Model file for the job. Use its own axes, mm. A direction names the side the tool comes from. Give positions to 0.01 mm unless a question says otherwise; leave off trailing zeros. Order: outer loops, then holes, each group sorted by start corner. A loop starts at its lowest first (then second) coordinate and runs counter-clockwise, first axis right, second up. Notation, with made-up numbers: (38, 48) - (68, 48) arc R13 cw to (68, 72) - close; hole circle Ø2 at (-27.5, 35). An arc over 180 degrees is marked (long way). Use CSV: the item, a comma, the result in double quotes. Start each with the question number.
(1) Probe L1, parallel to Z at x = 34.8, y = -4.25; L2, parallel to X at y = -2, z = 34. List the from-to ranges inside material, lowest first.
(2) Band-saw the part on B-B, the plane y = -56. Give the cut face in (x, z), then the cut area to 3 significant figures.
(3) Band-saw the part on A-A, the plane x = -34.8. Give the cut face in (y, z), then the cut area to 3 significant figures.
(4) Drop flat-ended pins along their axis: pin 1 Ø3 at (x, y) = (6, 28) entering from +Z; pin 2 Ø5.5 at (y, z) = (-56, 36) entering from +X; pin 3 Ø16 at (x, z) = (38, -38) entering from -Y. Give the stop position or say it passes through.
(5) Tool access for faces 1 (the flat face through (27.9, -45, -35)), 2 (the flat face through (-35, -45, -27.9)), 3 (the cylindrical face through (26.4, -44.51, 41.47)), 4 (the flat face through (-39, 0, 1)), 5 (the cylindrical face through (-26.4, -44.51, 41.47)): list every direction of +Z, -Z, +X, -X, +Y, -Y with a clear straight run to the whole face (end or side of a thin tool).
(6) Band-saw the part on C-C, the plane x = 0. Give the cut face in (y, z).
(7) Band-saw the part on D-D, the plane z = 34.8. Give the cut face in (x, y), then the cut area to 3 significant figures.
from build123d import *

# Parameters (mm, degrees)
F1_DEPTH  = 80
F2_W      = 15
F2_H      = 15
F3_DEPTH  = 70
F4_R      = 3.25
F5_DEPTH  = 10
F6_R      = 5
F7_R      = 36.5
F8_DEPTH  = 1.6
F9_R      = 7
F10_DEPTH = 35
F13_DEPTH = 5


with BuildPart() as f1:
    # F0 (on Front) → F1 (new body)
    with BuildSketch(Plane.XZ):
        with BuildLine():
            Line((37.9, 42.9), (-37.9, 42.9))
            ThreePointArc((-37.9, 42.9), (-41.4355339059, 41.4355339059), (-42.9, 37.9))
            Line((-42.9, 37.9), (-42.9, -37.9))
            ThreePointArc((-42.9, -37.9), (-41.4355339059, -41.4355339059), (-37.9, -42.9))
            Line((-37.9, -42.9), (37.9, -42.9))
            ThreePointArc((37.9, -42.9), (41.4355339059, -41.4355339059), (42.9, -37.9))
            Line((42.9, -37.9), (42.9, 37.9))
            ThreePointArc((42.9, 37.9), (41.4355339059, 41.4355339059), (37.9, 42.9))
        make_face()
    extrude(amount=F1_DEPTH)

    # F2 (on face) → F3 (cut)
    with BuildSketch(Plane.XZ.offset(80)):
        with Locations((35.4, 35.4)):
            Rectangle(F2_W, F2_H)
        with Locations((-35.4, 35.4)):
            Rectangle(F2_W, F2_H)
        with Locations((-35.4, -35.4)):
            Rectangle(F2_W, F2_H)
        with Locations((35.4, -35.4)):
            Rectangle(F2_W, F2_H)
    extrude(amount=-F3_DEPTH, mode=Mode.SUBTRACT)

    # F4 (on face) → F5 (cut, through all)
    with BuildSketch(Plane(origin=(0, 0, 0), x_dir=(-1, 0, 0), z_dir=(0, 1, 0))):
        with Locations((34.8, 34.8)):
            Circle(F4_R)
        with Locations((-34.8, 34.8)):
            Circle(F4_R)
        with Locations((34.8, -34.8)):
            Circle(F4_R)
        with Locations((-34.8, -34.8)):
            Circle(F4_R)
    extrude(amount=-F5_DEPTH, mode=Mode.SUBTRACT)

    # F6
    f6_edges = [f1.edges().sort_by_distance(p)[0] for p in [
        (-42.9, -45, 27.9),
        (-42.9, -45, -27.9),
        (-27.9, -45, -27.9),
        (-27.9, -45, -42.9),
        (27.9, -45, -42.9),
        (-27.9, -45, 42.9),
        (27.9, -45, -27.9),
        (42.9, -45, -27.9),
        (42.9, -45, 27.9),
        (27.9, -45, 42.9),
        (27.9, -45, 27.9),
        (-27.9, -45, 27.9),
    ]]
    fillet(f6_edges, radius=F6_R)

    # F7 (on face) → F8 (join)
    with BuildSketch(Plane(origin=(0, 0, 0), x_dir=(-1, 0, 0), z_dir=(0, 1, 0))):
        Circle(F7_R)
    extrude(amount=F8_DEPTH)

    # F9 (on face) → F10 (join)
    with BuildSketch(Plane(origin=(0, 0, 0), x_dir=(-1, 0, 0), z_dir=(0, 1, 0))):
        Circle(F9_R)
    extrude(amount=F10_DEPTH)

    # F12 (on offset) → F13 (cut)
    with BuildSketch(Plane.YZ.offset(4)):
        with BuildLine():
            Line((35, 2.5), (12.5, 2.5))
            ThreePointArc((12.5, 2.5), (10.732233047, 1.767766953), (10, 0))
            ThreePointArc((10, 0), (10.732233047, -1.767766953), (12.5, -2.5))
            Line((12.5, -2.5), (35, -2.5))
            Line((35, -2.5), (35, 0))
            Line((35, 0), (35, 2.5))
        make_face()
    extrude(amount=F13_DEPTH, mode=Mode.SUBTRACT)


solid = f1.part
Answer block:
1,L1,"z = -42.9 to -38.05, -31.55 to 31.55, 38.05 to 42.9"
1,L2,"x = -42.9 to -37.95, -31.65 to 31.65, 37.95 to 42.9"
2,outline,"(-42.9, -22.9) arc R5 ccw to (-37.9, -27.9) - (-32.9, -27.9) arc R5 cw to (-27.9, -32.9) - (-27.9, -37.9) arc R5 ccw to (-22.9, -42.9) - (22.9, -42.9) arc R5 ccw to (27.9, -37.9) - (27.9, -32.9) arc R5 cw to (32.9, -27.9) - (37.9, -27.9) arc R5 ccw to (42.9, -22.9) - (42.9, 22.9) arc R5 ccw to (37.9, 27.9) - (32.9, 27.9) arc R5 cw to (27.9, 32.9) - (27.9, 37.9) arc R5 ccw to (22.9, 42.9) - (-22.9, 42.9) arc R5 ccw to (-27.9, 37.9) - (-27.9, 32.9) arc R5 cw to (-32.9, 27.9) - (-37.9, 27.9) arc R5 ccw to (-42.9, 22.9) - close"
2,area,"6,440 mm2"
3,outline,"(-80, -27.9) - (-10, -27.9) - (-10, -31.55) - (0, -31.55) - (0, -11.01) - (1.6, -11.01) - (1.6, 11.01) - (0, 11.01) - (0, 31.55) - (-10, 31.55) - (-10, 27.9) - (-80, 27.9) - close; (-10, -42.9) - (0, -42.9) - (0, -38.05) - (-10, -38.05) - close; (-10, 38.05) - (0, 38.05) - (0, 42.9) - (-10, 42.9) - close"
3,area,"4,670 mm2"
4,pin 1,"stops at z = 5.36"
4,pin 2,"stops at x = 27.9"
4,pin 3,"stops at y = -10"
5,face 1,"-Z, +X, -Y"
5,face 2,"-Z, -X, -Y"
5,face 3,"+Z, +X, -Y"
5,face 4,"+Y"
5,face 5,"+Z, -X, -Y"
6,outline,"(-80, -42.9) - (0, -42.9) - (0, -36.5) - (1.6, -36.5) - (1.6, -7) - (35, -7) - (35, 7) - (1.6, 7) - (1.6, 36.5) - (0, 36.5) - (0, 42.9) - (-80, 42.9) - close"
7,outline,"(-42.9, -10) - (-38.05, -10) - (-38.05, 0) - (-42.9, 0) - close; (-31.55, -10) - (-27.9, -10) - (-27.9, -80) - (27.9, -80) - (27.9, -10) - (31.55, -10) - (31.55, 0) - (11.01, 0) - (11.01, 1.6) - (-11.01, 1.6) - (-11.01, 0) - (-31.55, 0) - close; (38.05, -10) - (42.9, -10) - (42.9, 0) - (38.05, 0) - close"
7,area,"4,670 mm2"
